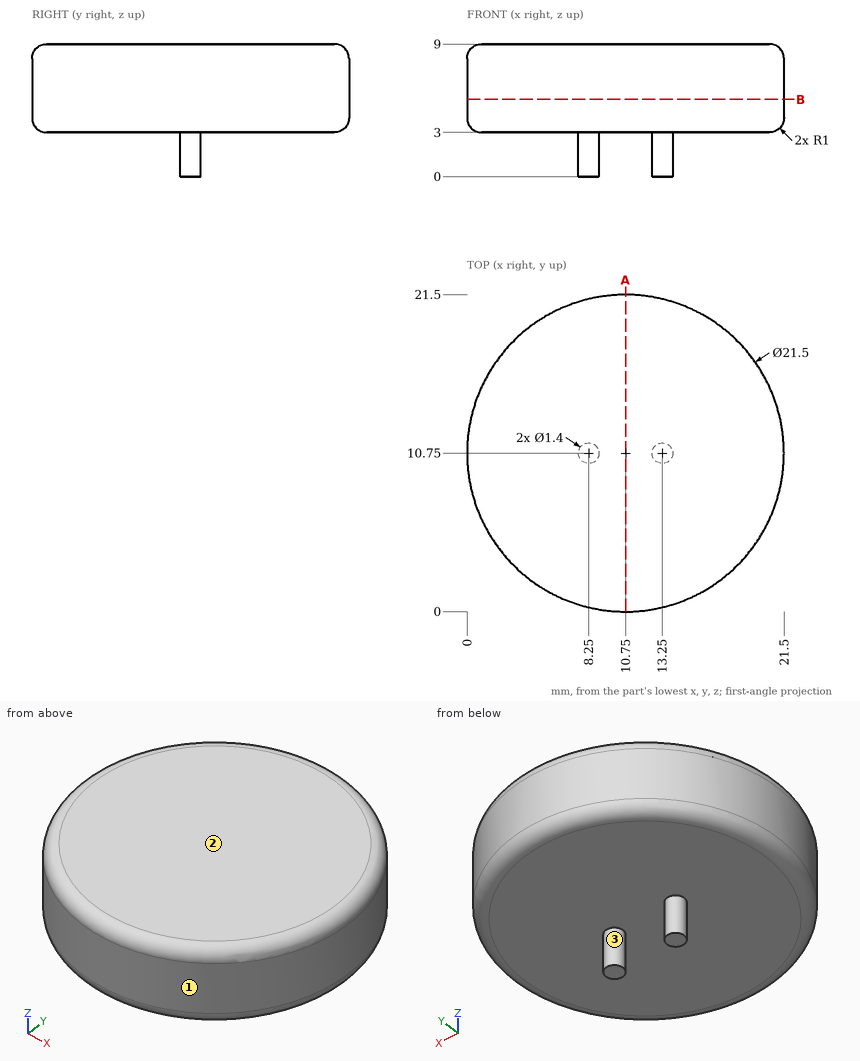
Could you check a few things on this drawing? It's one solid part, dimensions in mm from its lowest x, y, z. Give positions to 0.01 mm unless a question says otherwise; leave off trailing zeros. Write each loop counter-clockwise with the first axis right and the second up, starting at its lowest first coordinate (ties: lowest second). Pieces come first, ordered by that corner, then holes. Notation, with made-up numbers: (49.25, 55.5) -> (62.25, 55.5) arc R28 cw to (62.25, 93.5) -> close; hole circle Ø2 at (89, -31). An arc over 180 degrees is marked (long way). Answer as CSV lines item,"result". Start each with the question number.
(1) Please list where these lines run through material, in increasing order: line 1 (Z direction, x = 19.25, y = 14.25); line 2 (Y direction, x = 10.5, z = 5.25); line 3 (X direction, y = 4, z = 6.5).
(2) I'm going to push flat-ended pins straight in: pin 1 Ø3 at (x, y) = (16.5, 10.5) entering from -Z; pin 2 Ø5 at (y, z) = (6, 4.5) entering from +X; pin 3 Ø2 at (y, z) = (3.5, 3.5) entering from -X. Where does each tip first touch, or does it pass through?
(3) If we mould it in two halves opening along X, with no side actions, what happens to the marked faces 1, 2 and 3? For each: +X half, -X half, draft (parallel to the pull), parting line (faces both ways), or undercut.
(4) If we section it at B-B, the plane z = 5.25: Write out the boundary of the cut face in (x, y), and give its area (3 significant figures).
(5) If we section it at A-A, the plane x = 10.75: Write out the boundary of the cut face in (y, z), and give its area (3 significant figures).
Answer list:
1,line 1,"3 to 9"
1,line 2,"0 to 21.5"
1,line 3,"2.38 to 19.12"
2,pin 1,"z = 3"
2,pin 2,"x = 21.26"
2,pin 3,"x = 2.06"
3,face 1,"parting line"
3,face 2,"draft"
3,face 3,"undercut"
4,outline,"circle Ø21.5 at (10.75, 10.75)"
4,area,"363 mm^2"
5,outline,"(0, 4) arc R1 ccw to (1, 3) -> (20.5, 3) arc R1 ccw to (21.5, 4) -> (21.5, 8) arc R1 ccw to (20.5, 9) -> (1, 9) arc R1 ccw to (0, 8) -> close"
5,area,"128 mm^2"
